For this review, take the finished solid that the model builds, in its own axes (mm). Round coordinates to 2 decimals unless told otherwise and drop trailing zeros. Loops run counter-clockwise (first coordinate to the right, second up) from the corner with the lowest first, then second, coordinate; pieces in that order, holes last. Notation, with made-up numbers: M 7.25,-5 L 11.25,-5 A15 cw 11.25,20 Z; hole C 40.5,88 d6. An arc over 180 degrees is marked long. Write item = value, one per line. Start each with the question number.
```python
from build123d import *

# Parameters (mm, degrees)
SKETCH1_W           = 10
SKETCH1_H           = 20
BOSS_EXTRUDE1_DEPTH = 3
SKETCH2_R           = 2
CUT_EXTRUDE1_DEPTH  = 3
FILLET1_R           = 0.5


with BuildPart() as part:
    # Sketch1 → Boss-Extrude1 (new body)
    with BuildSketch(Plane(origin=(0, 0, 0), x_dir=(1, 0, 0), z_dir=(0, 1, 0))):
        Rectangle(SKETCH1_W, SKETCH1_H)
    extrude(amount=BOSS_EXTRUDE1_DEPTH)

    # Sketch2 → Cut-Extrude1 (cut)
    with BuildSketch(Plane(origin=(0, 3, 0), x_dir=(1, 0, 0), z_dir=(0, 1, 0))):
        with Locations(Location((0, -5.028947697, 0), (0, 0, 270))):
            Circle(SKETCH2_R)
    extrude(amount=-CUT_EXTRUDE1_DEPTH, mode=Mode.SUBTRACT)

    # Fillet1
    fillet1_edges = [part.edges().sort_by_distance(p)[0] for p in [
        (-5, 3, 0),
        (0, 3, 10),
        (5, 3, 0),
        (0, 3, -10),
    ]]
    fillet(fillet1_edges, radius=FILLET1_R)


solid = part.part
```
(1) Draft analysis for pull direction X (two halves, no side actions). For faces 1 (the cylindrical face through (-1.217, 1.521, 3.442)), 2 (the flat face through (0, 1, -10)), 3 (the flat face through (5, 1, 0)), state which applies: +X half, -X half, draft (parallel to the pull), parting line (faces both ways), or undercut.
(2) Wall thickness on L1, parallel to X at y = 0.75, z = 4; L2, parallel to X at y = 0.9, z = 5.75; L3, parallel to Z at x = -1.75, y = 0.45: over which ranges is each line inside the solid? List them lowest first.
(3) Add section B-B on y = 0.4. Write out the cut boundary in (x, z).
(4) Add section A-A on x = 0. Write out the cut boundary in (y, z).
Answer sheet:
q1.face_1 = undercut
q1.face_2 = draft
q1.face_3 = +X half
q2.L1 = -5 to -1.72, 1.72 to 5
q2.L2 = -5 to -1.87, 1.87 to 5
q2.L3 = -10 to 4.06, 6 to 10
q3.outline = M -5,-10 L 5,-10 L 5,10 L -5,10 Z; hole C 0,5.03 d4
q4.outline = M 0,-10 L 2.5,-10 A0.5 ccw 3,-9.5 L 3,3.03 L 0,3.03 Z; M 0,7.03 L 3,7.03 L 3,9.5 A0.5 ccw 2.5,10 L 0,10 Z
